from build123d import *

# Parameters (mm, degrees)
SKETCH_1_W               = 196
SKETCH_1_H               = 80
EXTRUDE_1_DEPTH          = 3
CUT_EXTRUDE_1_REACH      = 107.891
SKETCH_2_W               = 20
SKETCH_2_H               = 5
PATTERN_LINEAR_1_COUNT   = 3
PATTERN_LINEAR_1_PITCH   = 40
PATTERN_LINEAR_2_COUNT   = 3
PATTERN_LINEAR_2_PITCH   = 40
CUT_EXTRUDE_2_REACH      = 107.891
SKETCH_3_W               = 5
SKETCH_3_H               = 25
MIRROR_2_COPY_1_REACH    = 107.891
MIRROR_2_COPY_1_SKETCH_W = 20
MIRROR_2_COPY_1_SKETCH_H = 5
MIRROR_2_COPY_2_REACH    = 107.891
MIRROR_2_COPY_2_SKETCH_W = 20
MIRROR_2_COPY_2_SKETCH_H = 5
MIRROR_2_COPY_3_REACH    = 107.891
MIRROR_2_COPY_3_SKETCH_W = 20
MIRROR_2_COPY_3_SKETCH_H = 5
MIRROR_2_COPY_4_REACH    = 107.891
MIRROR_2_COPY_4_SKETCH_W = 20
MIRROR_2_COPY_4_SKETCH_H = 5
MIRROR_5_COPY_1_REACH    = 107.891
MIRROR_5_COPY_1_SKETCH_W = 5
MIRROR_5_COPY_1_SKETCH_H = 25


with BuildPart() as part:
    # 스케치1 → 보스-돌출1 (new body)
    with BuildSketch(Plane(origin=(0, 0, 0), x_dir=(1, 0, 0), z_dir=(0, 1, 0))):
        Rectangle(SKETCH_1_W, SKETCH_1_H)
    extrude(amount=EXTRUDE_1_DEPTH)

    # 스케치2 → 컷-돌출1 (cut, up to next)
    with BuildSketch(Plane(origin=(0, 3, 0), x_dir=(1, 0, 0), z_dir=(0, 1, 0)), mode=Mode.PRIVATE) as cut_extrude_1_sk1:
        with Locations((0, -37.5)):
            Rectangle(SKETCH_2_W, SKETCH_2_H)
    cut_extrude_1_tool1 = extrude(cut_extrude_1_sk1.sketch, amount=-CUT_EXTRUDE_1_REACH, mode=Mode.PRIVATE) & part.part
    cut_extrude_1 = cut_extrude_1_tool1.solids().sort_by_distance((0, 3, 37.5))[0]
    add(cut_extrude_1, mode=Mode.SUBTRACT)

    # 선형 패턴1: 컷-돌출1 ×3
    with Locations(*[(i * PATTERN_LINEAR_1_PITCH, 0, 0) for i in range(1, PATTERN_LINEAR_1_COUNT)]):
        add(cut_extrude_1, mode=Mode.SUBTRACT)

    # 선형 패턴2: 컷-돌출1 ×3
    with Locations(*[(-i * PATTERN_LINEAR_2_PITCH, 0, 0) for i in range(1, PATTERN_LINEAR_2_COUNT)]):
        add(cut_extrude_1, mode=Mode.SUBTRACT)

    # 스케치3 → 컷-돌출2 (cut, up to next)
    with BuildSketch(Plane(origin=(0, 3, 0), x_dir=(1, 0, 0), z_dir=(0, 1, 0)), mode=Mode.PRIVATE) as cut_extrude_2_sk1:
        with Locations((95.5, -22.5)):
            Rectangle(SKETCH_3_W, SKETCH_3_H)
    cut_extrude_2_tool1 = extrude(cut_extrude_2_sk1.sketch, amount=-CUT_EXTRUDE_2_REACH, mode=Mode.PRIVATE) & part.part
    cut_extrude_2 = cut_extrude_2_tool1.solids().sort_by_distance((95.5, 3, 22.5))[0]
    add(cut_extrude_2, mode=Mode.SUBTRACT)

    # 대칭 복사2: 컷-돌출1 across plane
    add(cut_extrude_1.mirror(Plane.XY), mode=Mode.SUBTRACT)

    # 대칭 복사2 copy 1 sketch → 대칭 복사2 copy 1 (cut, up to next)
    with BuildSketch(Plane(origin=(40, 3, 0), x_dir=(1, 0, 0), z_dir=(0, 1, 0)), mode=Mode.PRIVATE) as mirror_2_copy_1_sk1:
        with Locations((0, 37.5)):
            Rectangle(MIRROR_2_COPY_1_SKETCH_W, MIRROR_2_COPY_1_SKETCH_H)
    mirror_2_copy_1_tool1 = extrude(mirror_2_copy_1_sk1.sketch, amount=-MIRROR_2_COPY_1_REACH, mode=Mode.PRIVATE) & part.part
    add(mirror_2_copy_1_tool1.solids().sort_by_distance((40, 3, -37.5))[0], mode=Mode.SUBTRACT)

    # 대칭 복사2 copy 2 sketch → 대칭 복사2 copy 2 (cut, up to next)
    with BuildSketch(Plane(origin=(80, 3, 0), x_dir=(1, 0, 0), z_dir=(0, 1, 0)), mode=Mode.PRIVATE) as mirror_2_copy_2_sk1:
        with Locations((0, 37.5)):
            Rectangle(MIRROR_2_COPY_2_SKETCH_W, MIRROR_2_COPY_2_SKETCH_H)
    mirror_2_copy_2_tool1 = extrude(mirror_2_copy_2_sk1.sketch, amount=-MIRROR_2_COPY_2_REACH, mode=Mode.PRIVATE) & part.part
    add(mirror_2_copy_2_tool1.solids().sort_by_distance((80, 3, -37.5))[0], mode=Mode.SUBTRACT)

    # 대칭 복사2 copy 3 sketch → 대칭 복사2 copy 3 (cut, up to next)
    with BuildSketch(Plane(origin=(-40, 3, 0), x_dir=(1, 0, 0), z_dir=(0, 1, 0)), mode=Mode.PRIVATE) as mirror_2_copy_3_sk1:
        with Locations((0, 37.5)):
            Rectangle(MIRROR_2_COPY_3_SKETCH_W, MIRROR_2_COPY_3_SKETCH_H)
    mirror_2_copy_3_tool1 = extrude(mirror_2_copy_3_sk1.sketch, amount=-MIRROR_2_COPY_3_REACH, mode=Mode.PRIVATE) & part.part
    add(mirror_2_copy_3_tool1.solids().sort_by_distance((-40, 3, -37.5))[0], mode=Mode.SUBTRACT)

    # 대칭 복사2 copy 4 sketch → 대칭 복사2 copy 4 (cut, up to next)
    with BuildSketch(Plane(origin=(-80, 3, 0), x_dir=(1, 0, 0), z_dir=(0, 1, 0)), mode=Mode.PRIVATE) as mirror_2_copy_4_sk1:
        with Locations((0, 37.5)):
            Rectangle(MIRROR_2_COPY_4_SKETCH_W, MIRROR_2_COPY_4_SKETCH_H)
    mirror_2_copy_4_tool1 = extrude(mirror_2_copy_4_sk1.sketch, amount=-MIRROR_2_COPY_4_REACH, mode=Mode.PRIVATE) & part.part
    add(mirror_2_copy_4_tool1.solids().sort_by_distance((-80, 3, -37.5))[0], mode=Mode.SUBTRACT)

    # 대칭 복사3: 컷-돌출2 across plane
    add(cut_extrude_2.mirror(Plane(origin=(0, 0, 0), x_dir=(0, 0, 1), z_dir=(1, 0, 0))), mode=Mode.SUBTRACT)

    # 대칭 복사5: 컷-돌출2 across plane
    add(cut_extrude_2.mirror(Plane.XY), mode=Mode.SUBTRACT)

    # 대칭 복사5 copy 1 sketch → 대칭 복사5 copy 1 (cut, up to next)
    with BuildSketch(Plane(origin=(0, 3, 0), x_dir=(-1, 0, 0), z_dir=(0, 1, 0)), mode=Mode.PRIVATE) as mirror_5_copy_1_sk1:
        with Locations((95.5, -22.5)):
            Rectangle(MIRROR_5_COPY_1_SKETCH_W, MIRROR_5_COPY_1_SKETCH_H)
    mirror_5_copy_1_tool1 = extrude(mirror_5_copy_1_sk1.sketch, amount=-MIRROR_5_COPY_1_REACH, mode=Mode.PRIVATE) & part.part
    add(mirror_5_copy_1_tool1.solids().sort_by_distance((-95.5, 3, -22.5))[0], mode=Mode.SUBTRACT)


solid = part.part
Model file for the job. Use its own axes, mm. Round coordinates to 2 decimals unless told otherwise and drop trailing zeros. Loops run counter-clockwise (first coordinate to the right, second up) from the corner with the lowest first, then second, coordinate; pieces in that order, holes last.
1. Band-saw the part on A-A, the plane z = -30. List the corners of the cut face in (x, y).
Check values:
outline: (-93, 0) - (93, 0) - (93, 3) - (-93, 3) - close
2. Band-saw the part on B-B, the plane x = 37.5. List the corners of the cut face in (y, z).
Check values:
outline: (0, -35) - (3, -35) - (3, 35) - (0, 35) - close
3. Wall check: probe 1 along X at (y, z) = (2.35, -12); probe 2 along Z at (x, y) = (39.5, 1.25). Give the ranges that are in metal, low to high.
Check values:
probe 1: x = -93 to 93
probe 2: z = -35 to 35
4. Drop flat-ended pins along their axis: P1, Ø1.5, axis at x = 6, y = 2.5, coming from the +Z side; P2, Ø1.5, axis at y = 2, z = -18.5, coming from the -X side. Give the stop position or say it passes through.
Check values:
P1: stops at z = 35
P2: stops at x = -93
